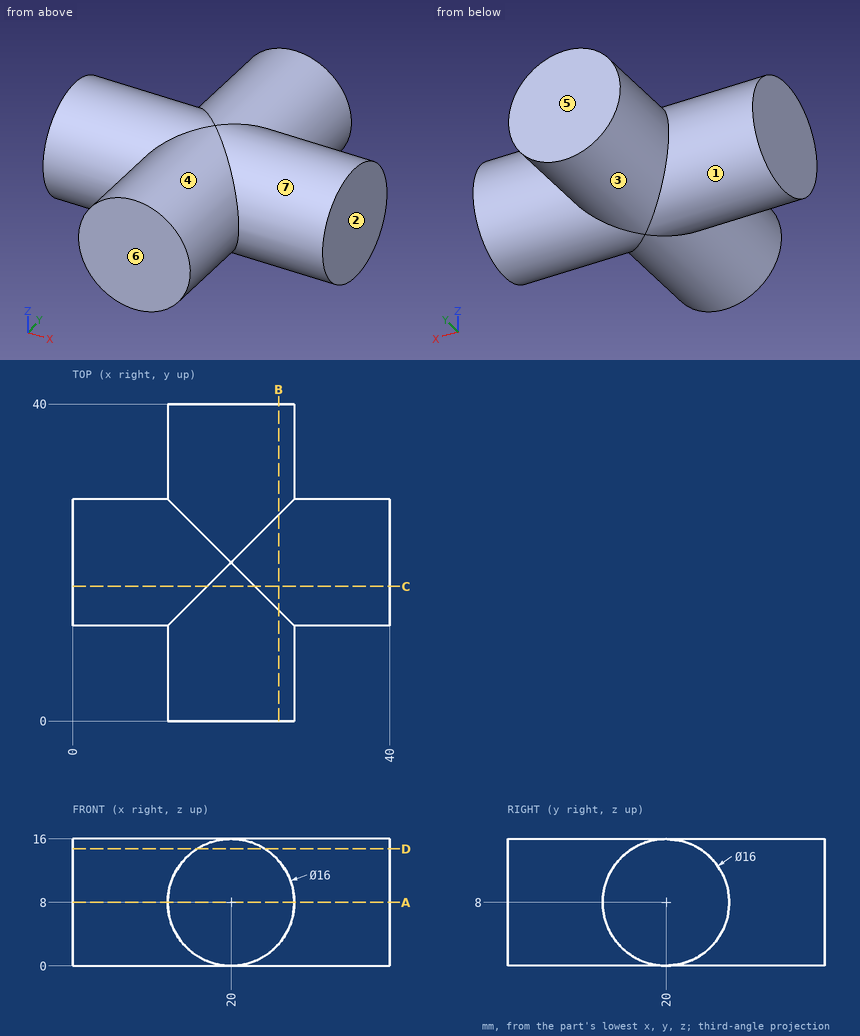
Can you work these out from the drawing? Everything is in mm from the part's minimum corner. A direction names the side the tool comes from. Coordinates: 2 decimals unless noted, no trailing zeros. Order: outer loops, then holes, each group sorted by start corner. A loop starts at its lowest first (then second) coordinate and runs counter-clockwise, first axis right, second up. Notation, with made-up numbers: (24.5, -27) -> (49.5, -27) arc R20 ccw to (49.5, 5) -> close; hole circle Ø9 at (50.5, 20). An arc over 180 degrees is marked (long way). Use one line per item in the form item = value.
Q1. Will these pins go through, and if not, where does the flat tip stop? P1, Ø1, axis at x = 28, z = 12, coming from the -Y side; P2, Ø3, axis at x = 12.5, y = 24, coming from the +Z side; P3, Ø8, axis at x = 7.5, z = 12, coming from the +Y side.
From the geometry:
P1 = 12.81
P2 = 15.6
P3 = 28
Q2. Which directions (+Z, -Z, +X, -X, +Y, -Y) give clear straight access to the entire face, cutting with the end or side of a thin tool? Please do the marked faces 1, 2, 3 and 4.
From the geometry:
face_1 = -X
face_2 = +Z, -Z, +X, +Y, -Y
face_3 = +Y
face_4 = -Y
Q3. Imagine slicing it at D-D, the plane z = 14.75. List the corners of the cut face in (x, y) for me, then the cut area to 3 significant figures.
From the geometry:
outline = (0, 15.71) -> (15.71, 15.71) -> (15.71, 0) -> (24.29, 0) -> (24.29, 15.71) -> (40, 15.71) -> (40, 24.29) -> (24.29, 24.29) -> (24.29, 40) -> (15.71, 40) -> (15.71, 24.29) -> (0, 24.29) -> close
area = 613 mm²
Q4. Imagine slicing it at C-C, the plane y = 17. List the corners of the cut face in (x, z) for me.
From the geometry:
outline = (0, 0.58) -> (17, 0.58) arc R8 ccw to (23, 0.58) -> (40, 0.58) -> (40, 15.42) -> (23, 15.42) arc R8 ccw to (17, 15.42) -> (0, 15.42) -> close
Q5. Imagine slicing it at A-A, the plane z = 8. List the corners of the cut face in (x, y) for me.
From the geometry:
outline = (0, 12) -> (12, 12) -> (12, 0) -> (28, 0) -> (28, 12) -> (40, 12) -> (40, 28) -> (28, 28) -> (28, 40) -> (12, 40) -> (12, 28) -> (0, 28) -> close
Q6. Imagine slicing it at B-B, the plane x = 26. List the corners of the cut face in (y, z) for me.
From the geometry:
outline = (0, 2.71) -> (14, 2.71) arc R8 ccw to (26, 2.71) -> (40, 2.71) -> (40, 13.29) -> (26, 13.29) arc R8 ccw to (14, 13.29) -> (0, 13.29) -> close
Q7. I need wall thicknesses on L1, parallel to Y at x = 28, z = 9.75; L2, parallel to X at y = 35, z = 8.5; L3, parallel to Y at x = 3.5, z = 14.5. Which ranges of each line are inside material? Lowest first, please.
From the geometry:
L1 = 12.19 to 27.81
L2 = 12.02 to 27.98
L3 = 15.34 to 24.66
Q8. We'd pull the mould along Y, two halves only. Please class the marked faces 5, 6 and 7: released by +Y, released by -Y, zero draft, split by the parting line, or undercut.
From the geometry:
face_5 = released by +Y
face_6 = released by -Y
face_7 = split by the parting line
